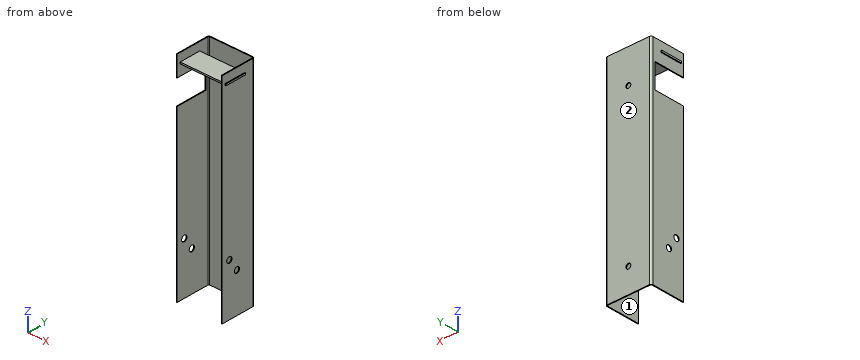
from build123d import *

# Parameters (mm, degrees)
BOSS_EXTRUDE1_DEPTH      = 261
FILLET1_R                = 2
FILLET2_R                = 1
BOSS_EXTRUDE2_DEPTH      = 56
BOSS_EXTRUDE2_DEPTH_BACK = 2
SKETCH2_W                = 2
SKETCH2_H                = 26
SKETCH3_R                = 3
CUT_EXTRUDE1_DEPTH       = 11
SKETCH4_W                = 30
SKETCH4_H                = 40
CUT_EXTRUDE2_DEPTH       = 10
SKETCH5_R                = 3.5
CUT_EXTRUDE3_DEPTH       = 69


with BuildPart() as part:
    # Sketch1 → Boss-Extrude1 (new body)
    with BuildSketch(Plane.XY):
        Polygon((27, -21.5), (27, -20.5), (27, 20.5), (-27, 20.5), (-27, -20.5), (-27, -21.5), (-28, -21.5), (-28, 21.5), (28, 21.5), (28, -21.5), align=None)
    extrude(amount=BOSS_EXTRUDE1_DEPTH)

    # Fillet1
    fillet1_edges = [part.edges().sort_by_distance(p)[0] for p in [
        (-28, 21.5, 130.5),
        (28, 21.5, 130.5),
    ]]
    fillet(fillet1_edges, radius=FILLET1_R)

    # Fillet2
    fillet2_edges = [part.edges().sort_by_distance(p)[0] for p in [
        (27, 20.5, 130.5),
        (-27, 20.5, 130.5),
    ]]
    fillet(fillet2_edges, radius=FILLET2_R)

    # Sketch2 → Boss-Extrude2 (add, two sides: drawn at the far end of the back side and taken through both)
    with BuildSketch(Plane(origin=(-27, 0, 0), x_dir=(0, 0, -1), z_dir=(1, 0, 0)).offset(-BOSS_EXTRUDE2_DEPTH_BACK)):
        with Locations((-250, -4.5)):
            Rectangle(SKETCH2_W, SKETCH2_H)
    extrude(amount=BOSS_EXTRUDE2_DEPTH + BOSS_EXTRUDE2_DEPTH_BACK)

    # Sketch3 → Cut-Extrude1 (cut)
    with BuildSketch(Plane(origin=(0, 21.5, 0), x_dir=(1, 0, 0), z_dir=(0, 1, 0))):
        with Locations(Location((0, -30, 0), (0, 0, 270))):
            Circle(SKETCH3_R)
        with Locations(Location((0, -220, 0), (0, 0, 270))):
            Circle(SKETCH3_R)
    extrude(amount=-CUT_EXTRUDE1_DEPTH, mode=Mode.SUBTRACT)

    # Sketch4 → Cut-Extrude2 (cut)
    with BuildSketch(Plane.ZY.offset(28)):
        with Locations((221, -3.5)):
            Rectangle(SKETCH4_W, SKETCH4_H)
    extrude(amount=-CUT_EXTRUDE2_DEPTH, mode=Mode.SUBTRACT)

    # Sketch5 → Cut-Extrude3 (cut)
    with BuildSketch(Plane.ZY.offset(28)):
        with Locations(Location((48, -2, 0), (0, 0, 270))):
            Circle(SKETCH5_R)
        with Locations(Location((63, -12, 0), (0, 0, 270))):
            Circle(SKETCH5_R)
    extrude(amount=-CUT_EXTRUDE3_DEPTH, mode=Mode.SUBTRACT)


solid = part.part
Build history of the part. All positions in model axes, mm. Face numbers are marked on the shaded views. Round coordinates to 2 decimals unless told otherwise and drop trailing zeros. Write each loop counter-clockwise with the first axis right and the second up, starting at its lowest first coordinate (ties: lowest second). Pieces come first, ordered by that corner, then holes. Notation, with made-up numbers: (42.25, -17) -> (64.25, -17) arc R11 ccw to (64.25, -4) -> close; hole circle Ø5 at (89, -27). An arc over 180 degrees is marked (long way). Use one line per item in the form item = value.
Q1. Band-saw the part on D-D, the plane x = 0. Write the cut outline in (y, z).
Conclusion:
outline = (-17.5, 249) -> (8.5, 249) -> (8.5, 251) -> (-17.5, 251) -> close; (20.5, 0) -> (21.5, 0) -> (21.5, 27) -> (20.5, 27) -> close; (20.5, 33) -> (21.5, 33) -> (21.5, 217) -> (20.5, 217) -> close; (20.5, 223) -> (21.5, 223) -> (21.5, 261) -> (20.5, 261) -> close
Q2. Band-saw the part on B-B, the plane x = -20. Write the cut outline in (y, z), then the cut area to 3 significant figures.
Conclusion:
outline = (-17.5, 249) -> (8.5, 249) -> (8.5, 251) -> (-17.5, 251) -> close; (20.5, 0) -> (21.5, 0) -> (21.5, 261) -> (20.5, 261) -> close
area = 313 mm²
Q3. Two-plate mould, pull along X, no slides. Class the marked faces 1 and 2: released by +X, released by -X, zero draft, split by the parting line, or undercut.
Conclusion:
face_1 = undercut
face_2 = zero draft
Q4. Band-saw the part on A-A, the plane z = 30. Write the cut outline in (x, y), then the cut area to 3 significant figures.
Conclusion:
outline = (-28, -21.5) -> (-27, -21.5) -> (-27, 19.5) arc R1 cw to (-26, 20.5) -> (-3, 20.5) -> (-3, 21.5) -> (-26, 21.5) arc R2 ccw to (-28, 19.5) -> close; (3, 20.5) -> (26, 20.5) arc R1 cw to (27, 19.5) -> (27, -21.5) -> (28, -21.5) -> (28, 19.5) arc R2 ccw to (26, 21.5) -> (3, 21.5) -> close
area = 133 mm²
Q5. Band-saw the part on C-C, the plane y = 12.5. Write the cut outline in (x, z).
Conclusion:
outline = (-28, 0) -> (-27, 0) -> (-27, 206) -> (-28, 206) -> close; (-28, 236) -> (-27, 236) -> (-27, 261) -> (-28, 261) -> close; (27, 0) -> (28, 0) -> (28, 261) -> (27, 261) -> close
Q6. Drill centre lines: L1, parallel to Z at x = -27.3, y = -2; L2, parallel to X at y = -6, z = 247; L3, parallel to Z at x = 27.75, y = -12. Where is each one in solid material? Low to high.
Conclusion:
L1 = 0 to 44.5, 51.5 to 206, 236 to 261
L2 = -28 to -27, 27 to 28
L3 = 0 to 59.5, 66.5 to 261
Q7. Drop flat-ended pins along their axis: P1, Ø5, axis at x = 14, y = -11, coming from the +Z side; P2, Ø0.5, axis at x = 28.5, y = -4, coming from the -Z side; P3, Ø4, axis at y = -15, z = 180, coming from the -X side. Give the stop position or say it passes through.
Conclusion:
P1 = 251
P2 = 249
P3 = -28
